For this review, take the finished solid that the model builds, in its own axes (mm). Face numbers are marked on the shaded views. A direction names the side the tool comes from. Round coordinates to 2 decimals unless told otherwise and drop trailing zeros. Loops run counter-clockwise (first coordinate to the right, second up) from the corner with the lowest first, then second, coordinate; pieces in that order, holes last.
1) Mouldability with a two-part tool opening along X and no side actions: class the marked faces 3, 4 and 5 as pulls with the +X half, pulls with the -X half, needs draft (parallel to the pull), parting line crosses it, or undercut.
2) Insertion check: pin 1 (11.5 mm diameter, centred on x = -1.78, y = 39.32, fed in from -Z). The pin has a flat end and moves straight along its axis. Give the tip position at first contact, or say it passes through.
3) Tool access review of the marked faces 1 and 2: name each direction out of +Z, -Z, +X, -X, +Y, -Y from which nothing blocks a thin tool from reaching the whole face with its end or side.
4) Take a section at A-A (y = 16.5). State the section outline as (x, z) points, then the cut area to 3 significant figures.
5) Take a section at B-B (x = 7.5). State the section outline as (y, z) points, then the cut area to 3 significant figures.
6) Wall thickness on L1, parallel to X at y = 12, z = 4; L2, parallel to Y at x = -2, z = 3; L3, parallel to X at y = 24.5, z = 2.5: over which ranges is each line inside the solid? List them lowest first.
7) Take a section at D-D (x = -3.5). State the section outline as (y, z) points.
8) Take a section at C-C (z = 2.5). State the section outline as (x, y) points (3 decimals), then the cut area to 3 significant figures.
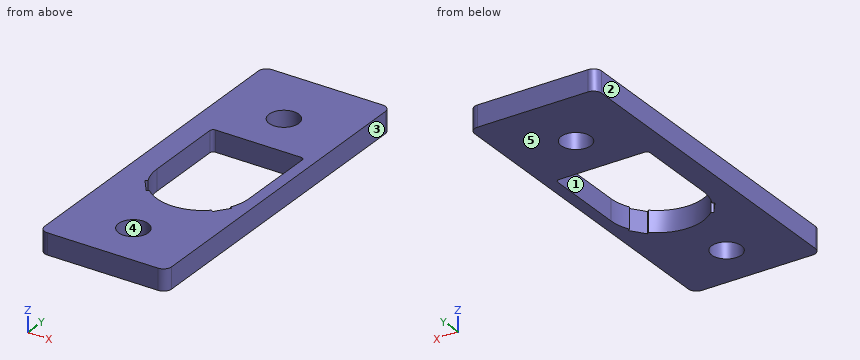
```python
from build123d import *

# Parameters (mm, degrees)
SKETCH1_W           = 38.1
SKETCH1_H           = 101.6
BOSS_EXTRUDE1_DEPTH = 6.35
CUT_EXTRUDE1_REACH  = 64.822
SKETCH2_R           = 4.445
FILLET5_R           = 1.016
FILLET6_R           = 2.46


with BuildPart() as part:
    # Sketch1 → Boss-Extrude1 (new body)
    with BuildSketch(Plane.XY):
        with Locations((-1.778, 8.128)):
            Rectangle(SKETCH1_W, SKETCH1_H)
        with BuildLine():
            Line((-13.843, 25.019), (-13.843, 0))
            ThreePointArc((-13.843, 0), (-13.476504522, -3.164249495), (-12.396424133, -6.16095104))
            Line((-12.396424133, -6.16095104), (-13.004984391, -6.619534088))
            Line((-13.004984391, -6.619534088), (-9.947764074, -10.676602479))
            Line((-9.947764074, -10.676602479), (-9.339203815, -10.218019431))
            ThreePointArc((-9.339203815, -10.218019431), (0, -13.843), (9.339203815, -10.218019431))
            Line((9.339203815, -10.218019431), (9.947764074, -10.676602479))
            Line((9.947764074, -10.676602479), (13.004984391, -6.619534088))
            Line((13.004984391, -6.619534088), (12.396424133, -6.16095104))
            ThreePointArc((12.396424133, -6.16095104), (13.476504522, -3.164249495), (13.843, 0))
            Line((13.843, 0), (13.843, 25.019))
            Line((13.843, 25.019), (-13.843, 25.019))
        make_face(mode=Mode.SUBTRACT)
    extrude(amount=BOSS_EXTRUDE1_DEPTH)

    # Sketch2 → Cut-Extrude1 (cut, up to next)
    with BuildSketch(Plane.XY.offset(6.35), mode=Mode.PRIVATE) as cut_extrude1_sk1:
        with Locations((-1.778, 39.322375)):
            Circle(SKETCH2_R)
    cut_extrude1_tool1 = extrude(cut_extrude1_sk1.sketch, amount=-CUT_EXTRUDE1_REACH, mode=Mode.PRIVATE) & part.part
    # Sketch2 → Cut-Extrude1 (cut, up to next)
    with BuildSketch(Plane.XY.offset(6.35), mode=Mode.PRIVATE) as cut_extrude1_sk2:
        with Locations((-1.778, -28.781375)):
            Circle(SKETCH2_R)
    cut_extrude1_tool2 = extrude(cut_extrude1_sk2.sketch, amount=-CUT_EXTRUDE1_REACH, mode=Mode.PRIVATE) & part.part
    add(cut_extrude1_tool1.solids().sort_by_distance((-1.778, 39.322375, 6.35))[0], mode=Mode.SUBTRACT)
    add(cut_extrude1_tool2.solids().sort_by_distance((-1.778, -28.781375, 6.35))[0], mode=Mode.SUBTRACT)

    # Fillet5
    fillet5_edges = [part.edges().sort_by_distance(p)[0] for p in [
        (13.843, 25.019, 3.175),
        (-13.843, 25.019, 3.175),
    ]]
    fillet(fillet5_edges, radius=FILLET5_R)

    # Fillet6
    fillet6_edges = [part.edges().sort_by_distance(p)[0] for p in [
        (-20.828, 58.928, 3.175),
        (17.272, 58.928, 3.175),
        (17.272, -42.672, 3.175),
        (-20.828, -42.672, 3.175),
    ]]
    fillet(fillet6_edges, radius=FILLET6_R)


solid = part.part
```
Response:
1. face 3: pulls with the +X half
1. face 4: undercut
1. face 5: needs draft
2. pin 1: stops at z = 0
3. face 1: +Z, -Z
3. face 2: +Z, -Z, -X, +Y, -Y
4. outline: (-20.83, 0) - (-13.84, 0) - (-13.84, 6.35) - (-20.83, 6.35) - close; (13.84, 0) - (17.27, 0) - (17.27, 6.35) - (13.84, 6.35) - close
4. area: 66.1 mm2
5. outline: (-42.67, 0) - (-11.64, 0) - (-11.64, 6.35) - (-42.67, 6.35) - close; (25.02, 0) - (58.93, 0) - (58.93, 6.35) - (25.02, 6.35) - close
5. area: 412 mm2
6. L1: x = -20.83 to -13.84, 13.84 to 17.27
6. L2: y = -42.67 to -33.22, -24.34 to -13.7, 25.02 to 34.88, 43.76 to 58.93
6. L3: x = -20.83 to -13.71, 13.71 to 17.27
7. outline: (-42.67, 0) - (-32.88, 0) - (-32.88, 6.35) - (-42.67, 6.35) - close; (-24.68, 0) - (-13.39, 0) - (-13.39, 6.35) - (-24.68, 6.35) - close; (25.02, 0) - (35.22, 0) - (35.22, 6.35) - (25.02, 6.35) - close; (43.42, 0) - (58.93, 0) - (58.93, 6.35) - (43.42, 6.35) - close
8. outline: (-20.828, -40.212) arc R2.46 ccw to (-18.368, -42.672) - (14.812, -42.672) arc R2.46 ccw to (17.272, -40.212) - (17.272, 56.468) arc R2.46 ccw to (14.812, 58.928) - (-18.368, 58.928) arc R2.46 ccw to (-20.828, 56.468) - close; hole (-13.843, 0) arc R13.843 ccw to (-12.396, -6.161) - (-13.005, -6.62) - (-9.948, -10.677) - (-9.339, -10.218) arc R13.843 ccw to (9.339, -10.218) - (9.948, -10.677) - (13.005, -6.62) - (12.396, -6.161) arc R13.843 ccw to (13.843, 0) - (13.843, 24.003) arc R1.016 ccw to (12.827, 25.019) - (-12.827, 25.019) arc R1.016 ccw to (-13.843, 24.003) - close; hole circle Ø8.89 at (-1.778, -28.781); hole circle Ø8.89 at (-1.778, 39.322)
8. area: 2,740 mm2
